Check sheet for the modelled part. Datum: model origin and axes. Units: mm. Face numbers are marked on the shaded views. A direction names the side the tool comes from. Round coordinates to 2 decimals unless told otherwise and drop trailing zeros. Write each loop counter-clockwise with the first axis right and the second up, starting at its lowest first coordinate (ties: lowest second). Pieces come first, ordered by that corner, then holes. Notation, with made-up numbers: M 60.5,19 L 93.5,19 A12 cw 93.5,33 Z; hole C 47,76.5 d1. An arc over 180 degrees is marked long. One line per item, written item: value.
from build123d import *

# Parameters (mm, degrees)
F0_W     = 1283
F0_H     = 874
F0_H_2   = 16
F1_DEPTH = 16
F2_DEPTH = 584
F3_DEPTH = 100
F4_W     = 1283
F4_H     = 16
F5_DEPTH = 150


with BuildPart() as f1:
    # F0 (on Front) → F1 (new body)
    with BuildSketch(Plane.XZ):
        with Locations((-657.5, 437)):
            Rectangle(F0_W, F0_H)
        with Locations((-657.5, 882)):
            Rectangle(F0_W, F0_H_2)
        Polygon((-16, 0), (0, 0), (0, 890), (-16, 890), (-16, 874), align=None)
        Polygon((-1315, 0), (-1299, 0), (-1299, 874), (-1299, 890), (-1315, 890), align=None)
    extrude(amount=-F1_DEPTH)

    # F0 (on Front) → F2 (join)
    with BuildSketch(Plane.XZ):
        Polygon((-1315, 0), (-1299, 0), (-1299, 874), (-1299, 890), (-1315, 890), align=None)
        Polygon((-16, 0), (0, 0), (0, 890), (-16, 890), (-16, 874), align=None)
    extrude(amount=F2_DEPTH)

    # F0 (on Front) → F3 (join)
    with BuildSketch(Plane.XZ):
        with Locations((-657.5, 882)):
            Rectangle(F0_W, F0_H_2)
    extrude(amount=F3_DEPTH)

    # F4 (on face) → F5 (join)
    with BuildSketch(Plane.XZ.offset(584)):
        with Locations((-657.5, 882)):
            Rectangle(F4_W, F4_H)
    extrude(amount=-F5_DEPTH)


solid = f1.part
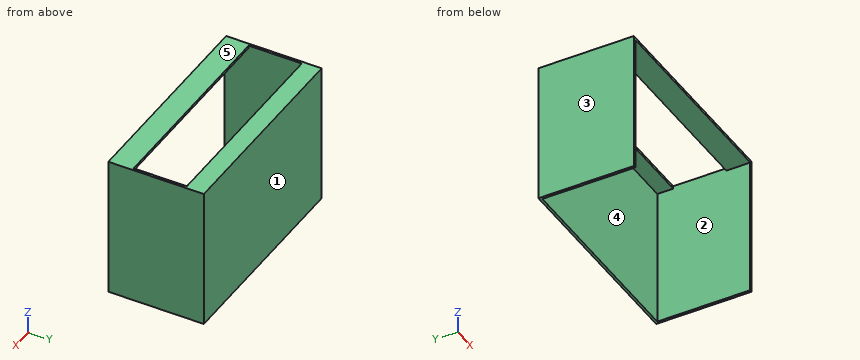
Q1. Draft check along X on the marked faces 1, 2 and 3. Enter one of: pulls with the +X half, pulls with the -X half, needs draft (parallel to the pull), parting line crosses it, or undercut.
Completed:
face 1: needs draft
face 2: undercut
face 3: pulls with the -X half
Q2. Depth check by flat-ended pin: P1, Ø3, axis at x = -1112, z = 562, coming from the -Y side. Enter the tip coordinate at first touch or a pass-through.
Completed:
P1: y = 0
Q3. Sectioned sample at D-D on y = -64. Enter the section's corners in (x, z).
Completed:
outline: M -1315,0 L -1299,0 L -1299,874 L -16,874 L -16,0 L 0,0 L 0,890 L -1315,890 Z
Q4. Sectioned sample at A-A on x = -100.5. Enter the section's corners in (y, z), and give its area (3 significant figures).
Completed:
outline: M -584,874 L -434,874 L -434,890 L -584,890 Z; M -100,874 L 0,874 L 0,0 L 16,0 L 16,890 L -100,890 Z
area: 18,200 mm^2
Q5. Scan lines: line 1 (X direction, y = -358, z = 561); line 2 (Z direction, x = -394, y = -63); line 3 (Y direction, x = -1077, z = 431). Record each from-to range of solid material in increasing order. Write a range as [from, to].
Completed:
line 1: [-1315, -1299], [-16, 0]
line 2: [874, 890]
line 3: [0, 16]
Q6. Sectioned sample at B-B on y = -316. Enter the section's corners in (x, z), and give its area (3 significant figures).
Completed:
outline: M -1315,0 L -1299,0 L -1299,890 L -1315,890 Z; M -16,0 L 0,0 L 0,890 L -16,890 Z
area: 28,500 mm^2
Q7. Sectioned sample at C-C on z = 636.5. Enter the section's corners in (x, y).
Completed:
outline: M -1315,-584 L -1299,-584 L -1299,0 L -16,0 L -16,-584 L 0,-584 L 0,16 L -1315,16 Z
Q8. Access from +Z, -Z, +X, -X, +Y, -Y to the whole of each face (thin tool, end or side, straight path). Record for the marked faces 4 and 5.
Completed:
face 4: -Z, -Y
face 5: +Z, +X, -X, +Y, -Y
